```python
from build123d import *

# Parameters (mm, degrees)
F0_R     = 2.5
F1_DEPTH = 3
F2_START = 3
F2_DEPTH = 3
F3_START = 3
F3_DEPTH = 6


# Not quite as in the source:
# - a feature names something its author has since deleted; it is built from what else it names


with BuildPart() as f1:
    # F0 (on Top) → F1 (new body)
    with BuildSketch(Plane.XY):
        with BuildLine():
            ThreePointArc((-10.5, 0), (0, -10.5), (10.5, 0))
            ThreePointArc((10.5, 0), (0, 10.5), (-10.5, 0))
        make_face()
        with BuildLine():
            Line((10.5, 9.237604307), (10.5, 6.7823299831))
            ThreePointArc((10.5, 6.7823299831), (11.9895788083, 3.5355339059), (12.5, 0))
            ThreePointArc((12.5, 0), (-3.5355339059, -11.9895788083), (-10.5, 6.7823299831))
            Line((-10.5, 6.7823299831), (-10.5, 9.237604307))
            ThreePointArc((-10.5, 9.237604307), (-14.5764952519, 3.9250122624), (-20.7631397208, 6.487604307))
            Line((-20.7631397208, 6.487604307), (-4.7631397208, -21.2252086141))
            ThreePointArc((-4.7631397208, -21.2252086141), (-1.4235047481, -13.1626165695), (5.5, -18.4752086141))
            ThreePointArc((5.5, -18.4752086141), (5.3125920446, -19.8987133621), (4.7631397208, -21.2252086141))
            Line((4.7631397208, -21.2252086141), (20.7631397208, 6.487604307))
            ThreePointArc((20.7631397208, 6.487604307), (14.5764952519, 3.9250122624), (10.5, 9.237604307))
        make_face()
        with BuildLine():
            ThreePointArc((16, 14.737604307), (12.1109127035, 13.1266916036), (10.5, 9.237604307))
            ThreePointArc((10.5, 9.237604307), (14.5764952519, 3.9250122624), (20.7631397208, 6.487604307))
            ThreePointArc((20.7631397208, 6.487604307), (21.3125920446, 7.814099559), (21.5, 9.237604307))
            ThreePointArc((21.5, 9.237604307), (19.8890872965, 13.1266916036), (16, 14.737604307))
        make_face()
        Polygon((11.3811978465, 9.237604307), (13.6905989232, 13.237604307), (18.3094010768, 13.237604307), (20.6188021535, 9.237604307), (18.3094010768, 5.237604307), (13.6905989232, 5.237604307), align=None, mode=Mode.SUBTRACT)
        with BuildLine():
            ThreePointArc((-20.7631397208, 6.487604307), (-14.5764952519, 3.9250122624), (-10.5, 9.237604307))
            ThreePointArc((-10.5, 9.237604307), (-12.1109127035, 13.1266916036), (-16, 14.737604307))
            ThreePointArc((-16, 14.737604307), (-20.7631397208, 11.987604307), (-20.7631397208, 6.487604307))
        make_face()
        Polygon((-18.3094010768, 13.237604307), (-13.6905989232, 13.237604307), (-11.3811978465, 9.237604307), (-13.6905989232, 5.237604307), (-18.3094010768, 5.237604307), (-20.6188021535, 9.237604307), align=None, mode=Mode.SUBTRACT)
        with BuildLine():
            ThreePointArc((-4.7631397208, -21.2252086141), (0, -23.9752086141), (4.7631397208, -21.2252086141))
            ThreePointArc((4.7631397208, -21.2252086141), (5.3125920446, -19.8987133621), (5.5, -18.4752086141))
            ThreePointArc((5.5, -18.4752086141), (-1.4235047481, -13.1626165695), (-4.7631397208, -21.2252086141))
        make_face()
        Polygon((-2.3094010768, -22.4752086141), (-4.6188021535, -18.4752086141), (-2.3094010768, -14.4752086141), (2.3094010768, -14.4752086141), (4.6188021535, -18.4752086141), (2.3094010768, -22.4752086141), align=None, mode=Mode.SUBTRACT)
        with BuildLine():
            Line((10.5, 6.7823299831), (10.5, 0))
            ThreePointArc((10.5, 0), (0, -10.5), (-10.5, 0))
            Line((-10.5, 0), (-10.5, 6.7823299831))
            ThreePointArc((-10.5, 6.7823299831), (-3.5355339059, -11.9895788083), (12.5, 0))
            ThreePointArc((12.5, 0), (11.9895788083, 3.5355339059), (10.5, 6.7823299831))
        make_face()
        with BuildLine():
            ThreePointArc((-10.5, 6.7823299831), (0, 12.5), (10.5, 6.7823299831))
            Line((10.5, 6.7823299831), (10.5, 9.237604307))
            Line((10.5, 9.237604307), (10.5, 14.737604307))
            Line((10.5, 14.737604307), (-10.5, 14.737604307))
            Line((-10.5, 14.737604307), (-10.5, 9.237604307))
            Line((-10.5, 9.237604307), (-10.5, 6.7823299831))
        make_face()
        Polygon((18.3094010768, 13.237604307), (13.6905989232, 13.237604307), (11.3811978465, 9.237604307), (13.6905989232, 5.237604307), (18.3094010768, 5.237604307), (20.6188021535, 9.237604307), align=None)
        with Locations((16, 9.237604307)):
            Circle(F0_R, mode=Mode.SUBTRACT)
        Polygon((-2.3094010768, -14.4752086141), (-4.6188021535, -18.4752086141), (-2.3094010768, -22.4752086141), (2.3094010768, -22.4752086141), (4.6188021535, -18.4752086141), (2.3094010768, -14.4752086141), align=None)
        with Locations((0, -18.4752086141)):
            Circle(F0_R, mode=Mode.SUBTRACT)
        Polygon((-11.3811978465, 9.237604307), (-13.6905989232, 13.237604307), (-18.3094010768, 13.237604307), (-20.6188021535, 9.237604307), (-18.3094010768, 5.237604307), (-13.6905989232, 5.237604307), align=None)
        with Locations((-16, 9.237604307)):
            Circle(F0_R, mode=Mode.SUBTRACT)
        with BuildLine():
            ThreePointArc((-10.5, 0), (0, 10.5), (10.5, 0))
            Line((10.5, 0), (10.5, 6.7823299831))
            ThreePointArc((10.5, 6.7823299831), (0, 12.5), (-10.5, 6.7823299831))
            Line((-10.5, 6.7823299831), (-10.5, 0))
        make_face()
        with BuildLine():
            Line((10.5, 14.737604307), (10.5, 9.237604307))
            ThreePointArc((10.5, 9.237604307), (12.1109127035, 13.1266916036), (16, 14.737604307))
            Line((16, 14.737604307), (10.5, 14.737604307))
        make_face()
        with BuildLine():
            ThreePointArc((-16, 14.737604307), (-12.1109127035, 13.1266916036), (-10.5, 9.237604307))
            Line((-10.5, 9.237604307), (-10.5, 14.737604307))
            Line((-10.5, 14.737604307), (-16, 14.737604307))
        make_face()
    extrude(amount=F1_DEPTH)

    # F0 (on Top) → F2 (join)
    with BuildSketch(Plane.XY.offset(F2_START)):
        with BuildLine():
            ThreePointArc((-20.7631397208, 6.487604307), (-14.5764952519, 3.9250122624), (-10.5, 9.237604307))
            ThreePointArc((-10.5, 9.237604307), (-12.1109127035, 13.1266916036), (-16, 14.737604307))
            ThreePointArc((-16, 14.737604307), (-20.7631397208, 11.987604307), (-20.7631397208, 6.487604307))
        make_face()
        Polygon((-18.3094010768, 13.237604307), (-13.6905989232, 13.237604307), (-11.3811978465, 9.237604307), (-13.6905989232, 5.237604307), (-18.3094010768, 5.237604307), (-20.6188021535, 9.237604307), align=None, mode=Mode.SUBTRACT)
        with BuildLine():
            ThreePointArc((-4.7631397208, -21.2252086141), (0, -23.9752086141), (4.7631397208, -21.2252086141))
            ThreePointArc((4.7631397208, -21.2252086141), (5.3125920446, -19.8987133621), (5.5, -18.4752086141))
            ThreePointArc((5.5, -18.4752086141), (-1.4235047481, -13.1626165695), (-4.7631397208, -21.2252086141))
        make_face()
        Polygon((-2.3094010768, -22.4752086141), (-4.6188021535, -18.4752086141), (-2.3094010768, -14.4752086141), (2.3094010768, -14.4752086141), (4.6188021535, -18.4752086141), (2.3094010768, -22.4752086141), align=None, mode=Mode.SUBTRACT)
        with BuildLine():
            ThreePointArc((16, 14.737604307), (12.1109127035, 13.1266916036), (10.5, 9.237604307))
            ThreePointArc((10.5, 9.237604307), (14.5764952519, 3.9250122624), (20.7631397208, 6.487604307))
            ThreePointArc((20.7631397208, 6.487604307), (21.3125920446, 7.814099559), (21.5, 9.237604307))
            ThreePointArc((21.5, 9.237604307), (19.8890872965, 13.1266916036), (16, 14.737604307))
        make_face()
        Polygon((11.3811978465, 9.237604307), (13.6905989232, 13.237604307), (18.3094010768, 13.237604307), (20.6188021535, 9.237604307), (18.3094010768, 5.237604307), (13.6905989232, 5.237604307), align=None, mode=Mode.SUBTRACT)
        with BuildLine():
            Line((10.5, 9.237604307), (10.5, 6.7823299831))
            ThreePointArc((10.5, 6.7823299831), (11.9895788083, 3.5355339059), (12.5, 0))
            ThreePointArc((12.5, 0), (-3.5355339059, -11.9895788083), (-10.5, 6.7823299831))
            Line((-10.5, 6.7823299831), (-10.5, 9.237604307))
            ThreePointArc((-10.5, 9.237604307), (-14.5764952519, 3.9250122624), (-20.7631397208, 6.487604307))
            Line((-20.7631397208, 6.487604307), (-4.7631397208, -21.2252086141))
            ThreePointArc((-4.7631397208, -21.2252086141), (-1.4235047481, -13.1626165695), (5.5, -18.4752086141))
            ThreePointArc((5.5, -18.4752086141), (5.3125920446, -19.8987133621), (4.7631397208, -21.2252086141))
            Line((4.7631397208, -21.2252086141), (20.7631397208, 6.487604307))
            ThreePointArc((20.7631397208, 6.487604307), (14.5764952519, 3.9250122624), (10.5, 9.237604307))
        make_face()
    extrude(amount=F2_DEPTH)

    # F0 (on Top) → F3 (join)
    with BuildSketch(Plane.XY.offset(F3_START)):
        with BuildLine():
            Line((10.5, 6.7823299831), (10.5, 0))
            ThreePointArc((10.5, 0), (0, -10.5), (-10.5, 0))
            Line((-10.5, 0), (-10.5, 6.7823299831))
            ThreePointArc((-10.5, 6.7823299831), (-3.5355339059, -11.9895788083), (12.5, 0))
            ThreePointArc((12.5, 0), (11.9895788083, 3.5355339059), (10.5, 6.7823299831))
        make_face()
    extrude(amount=F3_DEPTH)


solid = f1.part
```
Input: part model. Units: mm. Frame: model coordinates. A direction names the side the tool comes from. Give positions to 0.01 mm unless a question says otherwise; leave off trailing zeros. Order: outer loops, then holes, each group sorted by start corner. A loop starts at its lowest first (then second) coordinate and runs counter-clockwise, first axis right, second up. Notation, with made-up numbers: (88.5, 65) - (109.5, 65) arc R8 cw to (109.5, 79) - close; hole circle Ø11 at (85, -29.75). An arc over 180 degrees is marked (long way). Put each result on its own line as item: value.
Item 1: Section query C-C, the plane y = -7.5. Return loops of the section in (x, z), then the cut area to 3 significant figures.
Found:
outline: (-12.69, 0) - (12.69, 0) - (12.69, 6) - (10, 6) - (10, 9) - (7.35, 9) - (7.35, 3) - (-7.35, 3) - (-7.35, 9) - (-10, 9) - (-10, 6) - (-12.69, 6) - close
area: 124 mm^2
Item 2: Access query for faces 3 (the flat face through (0, -11, 9)), 4 (the flat face through (10.5, 5, 6)), 5 (the flat face through (-16, 5.238, 4)). Directions: +Z, -Z, +X, -X, +Y, -Y. A direction counts if a zero-diameter tool reaches every point of the face in a straight line with its end or side. Return the directions, or none.
Found:
face 3: +Z, +X, -X, +Y, -Y
face 4: +Z, +Y
face 5: +Z
Item 3: Section query B-B, the plane z = 4. Return loops of the section in (x, y).
Found:
outline: (-20.76, 6.49) - (-4.76, -21.23) arc R5.5 ccw to (4.76, -21.23) - (20.76, 6.49) arc R5.5 ccw (long way) to (10.5, 9.24) - (10.5, 0) arc R10.5 cw to (-10.5, 0) - (-10.5, 9.24) arc R5.5 ccw (long way) to start; hole (-20.62, 9.24) - (-18.31, 5.24) - (-13.69, 5.24) - (-11.38, 9.24) - (-13.69, 13.24) - (-18.31, 13.24) - close; hole (-4.62, -18.48) - (-2.31, -22.48) - (2.31, -22.48) - (4.62, -18.48) - (2.31, -14.48) - (-2.31, -14.48) - close; hole (11.38, 9.24) - (13.69, 5.24) - (18.31, 5.24) - (20.62, 9.24) - (18.31, 13.24) - (13.69, 13.24) - close
Item 4: Draft query along X for faces 1 (the flat face through (0, 2, 3)), 2 (the flat face through (0, 0, 0)). Return one class per face: +X half, -X half, draft (parallel to the pull), parting line (faces both ways), or undercut.
Found:
face 1: undercut
face 2: draft
Item 5: Section query D-D, the plane z = 8. Return loops of the section in (x, y).
Found:
outline: (-10.5, 0) - (-10.5, 6.78) arc R12.5 ccw (long way) to (10.5, 6.78) - (10.5, 0) arc R10.5 cw to start
Item 6: Contact query for flat-ended pins moving along their axis: pin 1 (2 mm diameter, centred on y = 2, z = 3.5, fed in from +X); pin 2 (1.5 mm diameter, centred on x = 0.5, z = 5, fed in from +Y); pin 3 (0.9 mm diameter, centred on x = 1, z = 5, fed in from -Y); pin 4 (4 mm diameter, centred on x = 17, y = -4.5, fed in from +Z). Output: stop coordinate, or through.
Found:
pin 1: stops at x = 18.75
pin 2: stops at y = -10.43
pin 3: stops at y = -23.95
pin 4: passes through
Item 7: Section query A-A, the plane x = 0. Return loops of the section in (y, z), then the cut area to 3 significant figures.
Found:
outline: (-23.98, 0) - (-20.98, 0) - (-20.98, 3) - (-22.48, 3) - (-22.48, 6) - (-23.98, 6) - close; (-15.98, 0) - (14.74, 0) - (14.74, 3) - (-10.5, 3) - (-10.5, 9) - (-12.5, 9) - (-12.5, 6) - (-14.48, 6) - (-14.48, 3) - (-15.98, 3) - close
area: 124 mm^2
Item 8: Ray query, L1, parallel to X at y = 9.5, z = 4.75; L2, parallel to X at y = 11.5, z = 5.5; L3, parallel to Z at x = 8, y = -13. Return the intervals inside material, ascending. Write a range as from..to.
Found:
L1: x = -21.49..-20.47, -11.53..-10.51, 10.51..11.53, 20.47..21.49
L2: x = -21.01..-19.31, -12.69..-10.99, 10.99..12.69, 19.31..21.01
L3: z = 0..6
